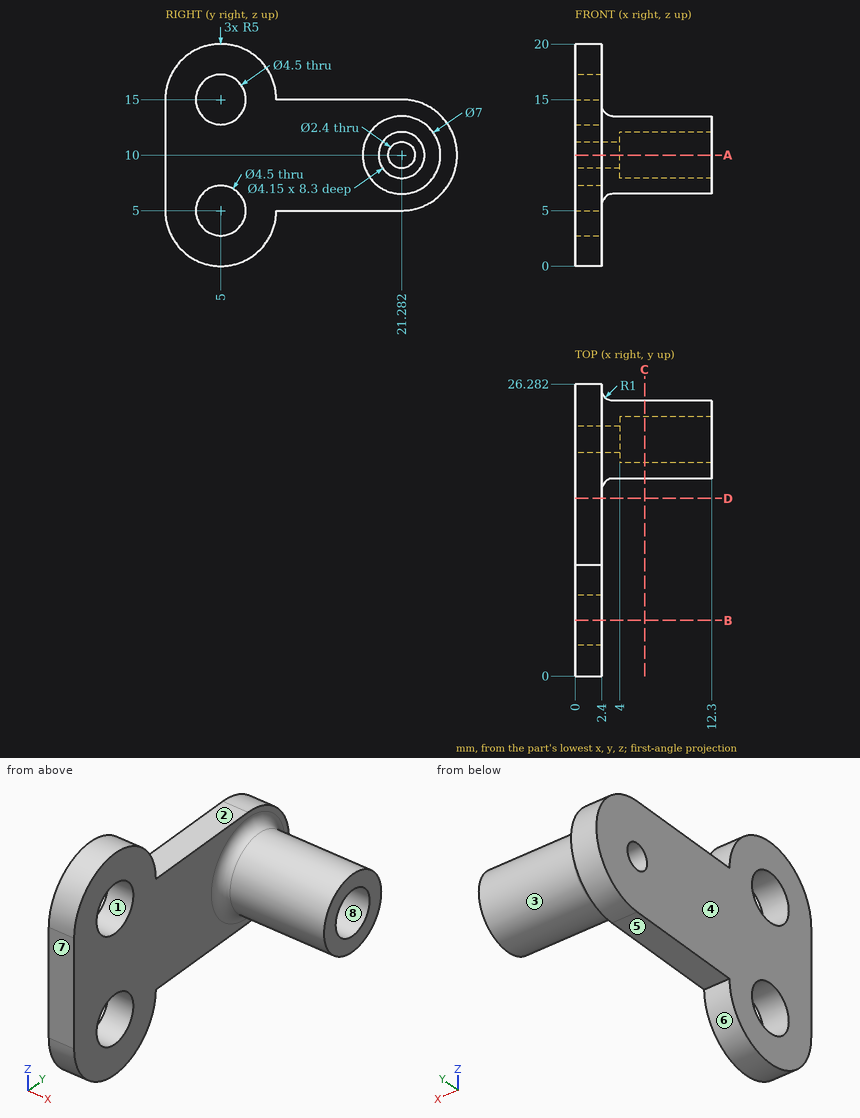
Source: three-view drawing plus pictorial views. Frame: mm from the lowest corner of the part. A direction names the side the tool comes from. Coordinates: 2 decimals unless noted, no trailing zeros. Order: outer loops, then holes, each group sorted by start corner. A loop starts at its lowest first (then second) coordinate and runs counter-clockwise, first axis right, second up.
Item 1: Cut plane B-B (y = 5). Return loops of the section in (x, z), plus the area to 3 significant figures.
Output values:
outline: (0, 0) - (2.4, 0) - (2.4, 2.75) - (0, 2.75) - close; (0, 7.25) - (2.4, 7.25) - (2.4, 12.75) - (0, 12.75) - close; (0, 17.25) - (2.4, 17.25) - (2.4, 20) - (0, 20) - close
area: 26.4 mm2
Item 2: Set-up query: the marked faces 1, 2, 3, 4 and 5. Return all of +Z, -Z, +X, -X, +Y, -Y with unobstructed straight access to the full face (end or side cutting, diameter ignored); none if empty.
Output values:
face 1: +X, -X
face 2: +Z, +X, -X, +Y
face 3: +X
face 4: +Z, -Z, -X, +Y, -Y
face 5: -Z, +X, -X, +Y
Item 3: Cut plane A-A (z = 10). Return loops of the section in (x, y).
Output values:
outline: (0, 0) - (2.4, 0) - (2.4, 16.78) arc R1 cw to (3.4, 17.78) - (12.3, 17.78) - (12.3, 19.21) - (4, 19.21) - (4, 20.08) - (0, 20.08) - close; (0, 22.48) - (4, 22.48) - (4, 23.36) - (12.3, 23.36) - (12.3, 24.78) - (3.4, 24.78) arc R1 cw to (2.4, 25.78) - (2.4, 26.28) - (0, 26.28) - close
Item 4: Cut plane D-D (y = 16). Return loops of the section in (x, z).
Output values:
outline: (0, 5) - (2.4, 5) - (2.4, 15) - (0, 15) - close
Item 5: First-contact query: P1, Ø6, axis at y = 14, z = 7, coming from the +X side; P2, Ø1.9, axis at x = 1.5, y = 18.5, coming from the -Z side; P3, Ø2, axis at y = 21.5, z = 10.5, coming from the +X side. Flat tips, straight axial feed; report the tip coordinate or a pass-through.
Output values:
P1: stops at x = 2.4
P2: stops at z = 5
P3: stops at x = 4
Item 6: Material intervals for line 1 (Y direction, x = 2.2, z = 10); line 2 (X direction, y = 7.25, z = 6.75); line 3 (Y direction, x = 9.5, z = 9.5), sorted ascending.
Output values:
line 1: y = 0 to 20.08, 22.48 to 26.28
line 2: x = 0 to 2.4
line 3: y = 17.82 to 19.27, 23.3 to 24.75
Item 7: Pull-direction query (Z, two-part tool) for the marked faces 6, 7 and 8; classes: pulls with the +Z half, pulls with the -Z half, needs draft (parallel to the pull), parting line crosses it, or undercut.
Output values:
face 6: pulls with the -Z half
face 7: needs draft
face 8: undercut
Item 8: Cut plane C-C (x = 6.25). Return loops of the section in (y, z) (3 decimals).
Output values:
outline: circle Ø7 at (21.282, 10); hole circle Ø4.15 at (21.282, 10)
